The model under review builds one solid part; all positions refer to its coordinate system, in mm. A direction names the side the tool comes from. Round coordinates to 2 decimals unless told otherwise and drop trailing zeros. Write each loop counter-clockwise with the first axis right and the second up, starting at its lowest first coordinate (ties: lowest second). Pieces come first, ordered by that corner, then holes. Notation, with made-up numbers: (58, 76.25) -> (79, 76.25) arc R32 ccw to (79, 114.25) -> close; hole circle Ø10 at (-36.5, 88). An arc over 180 degrees is marked (long way). Answer as a JSON object with one key per item and string values. Group by question number.
1) To check wall thickness, follow probe 1 along X at (y, z) = (0, 0.7); probe 2 along Z at (x, y) = (16, 10). State the ranges of each line that lie inside material, in increasing order. Write a range as [from, to].
2) Mouldability with a two-part tool opening along Y and no side actions: class faces 4 (the flat face through (-18, 0, 3)), 5 (the flat face through (-15, -3, 0)), 6 (the conical face through (-14.284, 14.602, 2.139)), 7 (the cylindrical face through (-0.66, -14.985, 0.493)) as pulls with the +Y half, pulls with the -Y half, needs draft (parallel to the pull), parting line crosses it, or undercut.
3) Machinability: for faces 1 (the flat face through (13, -8, 1)), 2 (the cylindrical face through (11.538, -11.795, 2.972)), 3 (the cylindrical face through (-11.538, 11.795, 2.972)), which of the approach directions +Z, -Z, +X, -X, +Y, -Y give a long, thin tool a straight path to every point of the face, cutting with its end or side? Answer none if there is none.
4) Insertion check: pin 1 Ø20 at (x, y) = (2.5, 1.5) entering from +Z; pin 2 Ø1.5 at (x, z) = (-1, 0.5) entering from -Y; pin 3 Ø2 at (y, z) = (-18.5, 3) entering from -X; pin 4 Ø1.2 at (y, z) = (19.5, 3) entering from +X. Each pin has a flat end and moves straight along its axis. Give the tip position at first contact, or say it passes through.
5) We need section A-A, the plane z = 2.8. Write out the cut boundary in (x, y) (3 decimals), then the cut area to 3 significant figures.
from build123d import *

# Parameters (mm, degrees)
F3_DEPTH = 4


with BuildPart() as f1:
    # F0 (on Right) → F1 (revolve)
    with BuildSketch(Plane.YZ):
        Polygon((15, 1), (15, 0), (20, 0), (20, 1), (21.5, 5), (16.5, 5), (16.5, 1), align=None)
    revolve(axis=Axis((0, 0, -1.199019), (0, 0, 1)))

    # F2 (on face) → F3 (cut)
    with BuildSketch(Plane.XY.offset(5)):
        with BuildLine():
            Line((0, -21.5), (0, -16.5))
            ThreePointArc((0, -16.5), (-11.667262, -11.667262), (-16.5, 0))
            Line((-16.5, 0), (-21.5, 0))
            ThreePointArc((-21.5, 0), (-15.202796, -15.202796), (0, -21.5))
        make_face()
        with BuildLine():
            Line((0, 21.5), (0, 16.5))
            ThreePointArc((0, 16.5), (11.667262, 11.667262), (16.5, 0))
            Line((16.5, 0), (21.5, 0))
            ThreePointArc((21.5, 0), (15.202796, 15.202796), (0, 21.5))
        make_face()
    extrude(amount=-F3_DEPTH, mode=Mode.SUBTRACT)


solid = f1.part
Here are the results:
{
 "1": {"probe 1": "x = [-20, -15], [15, 20]", "probe 2": "z = [0, 1]"},
 "2": {"face 4": "pulls with the -Y half", "face 5": "needs draft", "face 6": "pulls with the +Y half", "face 7": "undercut"},
 "3": {"face 1": "+Z", "face 2": "+Z, -X, +Y", "face 3": "+Z, +X, -Y"},
 "4": {"pin 1": "passes through", "pin 2": "stops at y = -20", "pin 3": "stops at x = 0", "pin 4": "stops at x = 0"},
 "5": {"outline": "(-20.675, 0) -> (-16.5, 0) arc R16.5 cw to (0, 16.5) -> (0, 20.675) arc R20.675 ccw to start; (0, -20.675) arc R20.675 ccw to (20.675, 0) -> (16.5, 0) arc R16.5 cw to (0, -16.5) -> close", "area": "244 mm^2"}
}
